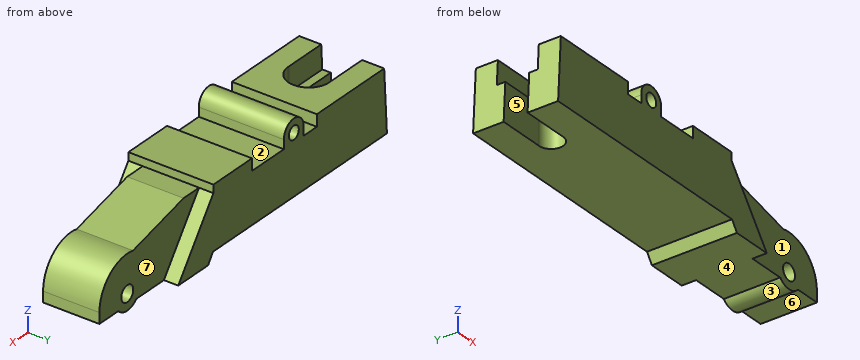
from build123d import *

# Parameters (mm, degrees)
F1_DEPTH  = 16
F2_R      = 1.5
F2_R_2    = 1.25
F3_DEPTH  = 16.001
F5_DEPTH  = 2.7
F8_DEPTH  = 14.501
F9_DEPTH  = 25
F11_DEPTH = 4.5


# Not quite as in the source:
# - a pattern or mirror of a feature is missing from the dataset's text; its kind, count and spacing are read off the source's solid


with BuildPart() as f1:
    # F0 (on Front) → F1 (new body)
    with BuildSketch(Plane.XZ):
        with BuildLine():
            Line((0.6909776407, 11.7), (0, 0))
            Line((0, 0), (43.7, 0))
            Line((43.7, 0), (44.92, -1.8))
            Line((44.92, -1.8), (59.3839320225, -1.8))
            ThreePointArc((59.3839320225, -1.8), (61.62, -2.8), (63.8560679775, -1.8))
            Line((63.8560679775, -1.8), (68.62, -1.8))
            Line((68.62, -1.8), (68.62, 0.2))
            ThreePointArc((68.62, 0.2), (66.0308120163, 5.6355070929), (60.1786464695, 7.05))
            Line((60.1786464695, 7.05), (47.4909776407, 10.2))
            Line((47.4909776407, 10.2), (43.5909776407, 10.2))
            Line((43.5909776407, 10.2), (43.5909776407, 11.7))
            Line((43.5909776407, 11.7), (33.8909776407, 11.7))
            Line((33.8909776407, 11.7), (33.8909776407, 9.5))
            Line((33.8909776407, 9.5), (25.8909776407, 9.5))
            Line((25.8909776407, 9.5), (25.8909776407, 11.2))
            ThreePointArc((25.8909776407, 11.2), (23.2847799515, 13.6977433917), (20.9, 10.9877963389))
            Line((20.9, 10.9877963389), (20.9, 9.5))
            Line((20.9, 9.5), (17.6, 9.5))
            Line((17.6, 9.5), (17.6, 11.7))
            Line((17.6, 11.7), (0.6909776407, 11.7))
        make_face()
    extrude(amount=F1_DEPTH)

    # F2 (on face) → F3 (cut, through all)
    with BuildSketch(Plane.XZ.offset(16)):
        with Locations((61.62, 0.2)):
            Circle(F2_R)
        with Locations((23.3909776407, 11.2)):
            Circle(F2_R_2)
    extrude(amount=-F3_DEPTH, mode=Mode.SUBTRACT)

    # F4 (on face) → F5 (cut)
    with BuildSketch(Plane.XZ.offset(16)):
        Polygon((69.0573006868, 10.2), (43.5909776407, 10.2), (52.42, -1.8), (58.7147176266, -4.3849991634), (70.332378149, -4.3849991634), align=None)
    f5 = extrude(amount=-F5_DEPTH, mode=Mode.SUBTRACT)

    # F5_copies: F5 across plane
    add(f5.mirror(Plane.ZX.offset(-8)), mode=Mode.SUBTRACT)

    # F7 (on face) → F8 (cut, through all)
    with BuildSketch(Plane.XY.offset(11.7)):
        with BuildLine():
            Line((8.9409776407, -5.75), (0.6909776407, -5.75))
            Line((0.6909776407, -5.75), (0.6909776407, -10.25))
            Line((0.6909776407, -10.25), (8.9409776407, -10.25))
            ThreePointArc((8.9409776407, -10.25), (11.1909776407, -8), (8.9409776407, -5.75))
        make_face()
    extrude(amount=-F8_DEPTH, mode=Mode.SUBTRACT)

    # F7 (on face) → F9 (cut)
    with BuildSketch(Plane.XY.offset(11.7)):
        with BuildLine():
            Line((8.9409776407, -5.75), (0.6909776407, -5.75))
            Line((0.6909776407, -5.75), (-0.8989692941, -5.75))
            Line((-0.8989692941, -5.75), (-0.8989692941, -10.25))
            Line((-0.8989692941, -10.25), (0.6909776407, -10.25))
            Line((0.6909776407, -10.25), (8.9409776407, -10.25))
            ThreePointArc((8.9409776407, -10.25), (11.1909776407, -8), (8.9409776407, -5.75))
        make_face()
    extrude(amount=-F9_DEPTH, mode=Mode.SUBTRACT)

    # F10 (on face) → F11 (cut)
    with BuildSketch(Plane.XY.offset(11.7)):
        with BuildLine():
            ThreePointArc((9.0590238842, -11.8481898452), (11.7047592925, -10.6803005393), (12.7909776407, -8))
            ThreePointArc((12.7909776407, -8), (11.7048621847, -5.3198055617), (9.0593193409, -4.1518192296))
            Line((9.0593193409, -4.1518192296), (8.8226359404, -4.1518192296))
            ThreePointArc((8.8226359404, -4.1518192296), (5.0909776435, -8.000147798), (8.8229313971, -11.8481898452))
            Line((8.8229313971, -11.8481898452), (9.0590238842, -11.8481898452))
        make_face()
        with BuildLine():
            Line((8.8226359404, -4.1518192296), (9.0593193409, -4.1518192296))
            ThreePointArc((9.0593193409, -4.1518192296), (8.9409776407, -4.15), (8.8226359404, -4.1518192296))
        make_face()
        with BuildLine():
            ThreePointArc((8.8229313971, -11.8481898452), (8.9409776407, -11.85), (9.0590238842, -11.8481898452))
            Line((9.0590238842, -11.8481898452), (8.8229313971, -11.8481898452))
        make_face()
        with BuildLine():
            ThreePointArc((8.8229313971, -11.8481898452), (5.0909776435, -8.000147798), (8.8226359404, -4.1518192296))
            Line((8.8226359404, -4.1518192296), (-1.5180813544, -4.1518192296))
            Line((-1.5180813544, -4.1518192296), (-2.6164921116, -11.8481898452))
            Line((-2.6164921116, -11.8481898452), (8.8229313971, -11.8481898452))
        make_face()
    extrude(amount=-F11_DEPTH, mode=Mode.SUBTRACT)


solid = f1.part
Work out the finished part from the listing and answer in its coordinate system (mm). Face numbers are marked on the shaded views. A direction names the side the tool comes from. Give positions to 0.01 mm unless a question says otherwise; leave off trailing zeros. Loops run counter-clockwise (first coordinate to the right, second up) from the corner with the lowest first, then second, coordinate; pieces in that order, holes last. Notation, with made-up numbers: (58, 35) - (89, 35) arc R27 cw to (89, 74) - close; hole circle Ø2 at (-2.75, -23). An arc over 180 degrees is marked (long way). Answer in a Markdown table with one row per item.
(1) Section D-D (y = -8.75) is taken. Give the vertices of the cut face in (x, z), and give its area (3 significant figures).
Results list:
| item | result |
|---|---|
| outline | (11.06, 0) - (43.7, 0) - (44.92, -1.8) - (59.38, -1.8) arc R3 ccw to (63.86, -1.8) - (68.62, -1.8) - (68.62, 0.2) arc R7 ccw to (60.18, 7.05) - (47.49, 10.2) - (43.59, 10.2) - (43.59, 11.7) - (33.89, 11.7) - (33.89, 9.5) - (25.89, 9.5) - (25.89, 11.2) arc R2.5 ccw (long way) to (20.9, 10.99) - (20.9, 9.5) - (17.6, 9.5) - (17.6, 11.7) - (12.72, 11.7) - (12.72, 7.2) - (11.06, 7.2) - close; hole circle Ø2.5 at (23.39, 11.2); hole circle Ø3 at (61.62, 0.2) |
| area | 590 mm² |
(2) Consider L1, parallel to Z at x = 23.5, y = -13.75; L2, parallel to Y at x = 5, z = 10.5; L3, parallel to Z at x = 61.62, y = -6.5. Determine where each line is inside the solid, lowest interval first. Write a range as [from, to].
Results list:
| item | result |
|---|---|
| L1 | z = [0, 9.95], [12.45, 13.7] |
| L2 | y = [-16, -11.85], [-4.15, 0] |
| L3 | z = [-2.8, -1.3], [1.7, 7.2] |
(3) Section A-A (y = -14) is taken. Give the vertices of the cut face in (x, z), and give its area (3 significant figures).
Results list:
| item | result |
|---|---|
| outline | (0, 0) - (43.7, 0) - (44.92, -1.8) - (52.42, -1.8) - (43.59, 10.2) - (43.59, 11.7) - (33.89, 11.7) - (33.89, 9.5) - (25.89, 9.5) - (25.89, 11.2) arc R2.5 ccw (long way) to (20.9, 10.99) - (20.9, 9.5) - (17.6, 9.5) - (17.6, 11.7) - (0.69, 11.7) - close; hole circle Ø2.5 at (23.39, 11.2) |
| area | 535 mm² |
(4) Section C-C (z = 4) is taken. Give the vertices of the cut face in (x, y), and give its area (3 significant figures).
Results list:
| item | result |
|---|---|
| outline | (0.24, -16) - (48.15, -16) - (48.15, -13.3) - (67.5, -13.3) - (67.5, -2.7) - (48.15, -2.7) - (48.15, 0) - (0.24, 0) - (0.24, -5.75) - (8.94, -5.75) arc R2.25 cw to (8.94, -10.25) - (0.24, -10.25) - close |
| area | 925 mm² |
(5) For a pull along X with two mould halves and no side action, classify the marked faces 1, 2 and 3 as pulls with the +X half, pulls with the -X half, needs draft (parallel to the pull), parting line crosses it, or undercut.
Results list:
| item | result |
|---|---|
| face 1 | needs draft |
| face 2 | undercut |
| face 3 | parting line crosses it |
(6) A tool of negligible diameter and unlimited length cuts with its end or side. For the marked faces 4, 5, 6 and 7, from which of +Z, -Z, +X, -X, +Y, -Y can it reach the whole face along a straight path? Write none if from no direction.
Results list:
| item | result |
|---|---|
| face 4 | -Z, -X, +Y, -Y |
| face 5 | +Z, -Z, -X |
| face 6 | -Z, +X, +Y, -Y |
| face 7 | +Z, +X, +Y |
(7) Flat-ended cylindrical pins translate along their axes: pin 1 Ø2.5 at (x, y) = (28, -10.5) entering from +Z; pin 2 Ø5 at (x, y) = (12.5, -11) entering from +Z; pin 3 Ø2 at (y, z) = (-3, 10) entering from -X; pin 4 Ø2 at (x, z) = (4, 5) entering from +Y. Find the tip coordinate at first contact, or state that the pin passes through.
Results list:
| item | result |
|---|---|
| pin 1 | stops at z = 9.5 |
| pin 2 | stops at z = 11.7 |
| pin 3 | stops at x = 0.53 |
| pin 4 | stops at y = 0 |
(8) Section B-B (x = 61.62) is taken. Give the vertices of the cut face in (y, z).
Results list:
| item | result |
|---|---|
| outline | (-13.3, -2.8) - (-2.7, -2.8) - (-2.7, -1.3) - (-13.3, -1.3) - close; (-13.3, 1.7) - (-2.7, 1.7) - (-2.7, 7.2) - (-13.3, 7.2) - close |
